Check sheet for the modelled part. Datum: model origin and axes. Units: mm. Round coordinates to 2 decimals unless told otherwise and drop trailing zeros. Loops run counter-clockwise (first coordinate to the right, second up) from the corner with the lowest first, then second, coordinate; pieces in that order, holes last. Notation, with made-up numbers: (77, -1) - (136, -1) arc R21 ccw to (136, 5) - close; hole circle Ø3 at (63, 63.25). An arc over 180 degrees is marked (long way). Put each result on its own line as item: value. Start each with the question number.
Item 1: Material ranges on line 1 along Y through (x, z) = (0, 3.75) (3 decimals); line 2 along Y through (x, z) = (7, 6); line 3 along X through (y, z) = (6.5, 0.5), recorded low to high.
Item 2: Section check D-D, the plane x = 0. Give the number of separate pieces and of enclosed holes in the cut face, and give its area (3 significant figures).
Item 3: Section check A-A, the plane z = 3.75. Record the cut outline in (x, y) (3 decimals), and give its area (3 significant figures).
Item 4: Section check C-C, the plane y = 58.72. Record the cut outline in (x, z), and give its area (3 significant figures).
Item 5: Section check B-B, the plane y = 0. Record the cut outline in (x, z) (3 decimals), and give its area (3 significant figures).
Item 6: Gauge pin test, flat end, axial feed: pin 1 Ø1.5 at (x, y) = (-7, 0) entering from +Z. Record the tip position at first contact, or that the pin passes through.
from build123d import *

# Parameters (mm, degrees)
F0_W     = 40
F0_H     = 100
F0_R     = 1.25
F0_R_2   = 1.525
F1_DEPTH = 8
F2_DEPTH = 7
F3_DEPTH = 5
F4_SIZE  = 0.99999


# Not quite as in the source:
# - a fillet or chamfer is up to 0.001 mm smaller than in the source, because OpenCascade refuses the exact size


with BuildPart() as f1:
    # F0 (on Top) → F1 (new body)
    with BuildSketch(Plane.XY):
        with Locations((0, 30)):
            Rectangle(F0_W, F0_H)
        with Locations((-7, 0)):
            Circle(F0_R, mode=Mode.SUBTRACT)
        Circle(F0_R_2, mode=Mode.SUBTRACT)
        with Locations((7, 0)):
            Circle(F0_R, mode=Mode.SUBTRACT)
        with BuildLine():
            ThreePointArc((-10.75, 30), (-10.1642135624, 31.4142135624), (-8.75, 32))
            Line((-8.75, 32), (8.75, 32))
            ThreePointArc((8.75, 32), (10.1642135624, 31.4142135624), (10.75, 30))
            Line((10.75, 30), (10.75, 11.6))
            Line((10.75, 11.6), (10.75, 5.5))
            ThreePointArc((10.75, 5.5), (8.75, 3.5), (6.75, 5.5))
            Line((6.75, 5.5), (-6.75, 5.5))
            ThreePointArc((-6.75, 5.5), (-8.75, 3.5), (-10.75, 5.5))
            Line((-10.75, 5.5), (-10.75, 11.6))
            Line((-10.75, 11.6), (-10.75, 30))
        make_face(mode=Mode.SUBTRACT)
        with BuildLine():
            Line((-1.53, 57.72), (-1.53, 59.72))
            ThreePointArc((-1.53, 59.72), (0, 61.25), (1.53, 59.72))
            Line((1.53, 59.72), (1.53, 57.72))
            ThreePointArc((1.53, 57.72), (0, 56.19), (-1.53, 57.72))
        make_face(mode=Mode.SUBTRACT)
        with Locations((7, 58.72)):
            Circle(F0_R, mode=Mode.SUBTRACT)
        with BuildLine():
            Line((8.75, 32), (-8.75, 32))
            ThreePointArc((-8.75, 32), (-10.1642135624, 31.4142135624), (-10.75, 30))
            Line((-10.75, 30), (-10.75, 11.6))
            ThreePointArc((-10.75, 11.6), (-10.1642135624, 10.1857864376), (-8.75, 9.6))
            Line((-8.75, 9.6), (8.75, 9.6))
            ThreePointArc((8.75, 9.6), (10.1642135624, 10.1857864376), (10.75, 11.6))
            Line((10.75, 11.6), (10.75, 30))
            ThreePointArc((10.75, 30), (10.1642135624, 31.4142135624), (8.75, 32))
        make_face()
        with BuildLine():
            ThreePointArc((-6, 26.3), (-5.4142135624, 27.7142135624), (-4, 28.3))
            Line((-4, 28.3), (4, 28.3))
            ThreePointArc((4, 28.3), (5.4142135624, 27.7142135624), (6, 26.3))
            Line((6, 26.3), (6, 15.3))
            ThreePointArc((6, 15.3), (5.4142135624, 13.8857864376), (4, 13.3))
            Line((4, 13.3), (-4, 13.3))
            ThreePointArc((-4, 13.3), (-5.4142135624, 13.8857864376), (-6, 15.3))
            Line((-6, 15.3), (-6, 26.3))
        make_face(mode=Mode.SUBTRACT)
        with BuildLine():
            ThreePointArc((-8.75, 9.6), (-10.1642135624, 10.1857864376), (-10.75, 11.6))
            Line((-10.75, 11.6), (-10.75, 5.5))
            ThreePointArc((-10.75, 5.5), (-8.75, 3.5), (-6.75, 5.5))
            Line((-6.75, 5.5), (6.75, 5.5))
            ThreePointArc((6.75, 5.5), (8.75, 3.5), (10.75, 5.5))
            Line((10.75, 5.5), (10.75, 11.6))
            ThreePointArc((10.75, 11.6), (10.1642135624, 10.1857864376), (8.75, 9.6))
            Line((8.75, 9.6), (-8.75, 9.6))
        make_face()
    extrude(amount=F1_DEPTH)

    # F0 (on Top) → F2 (cut)
    with BuildSketch(Plane.XY):
        with BuildLine():
            Line((8.75, 32), (-8.75, 32))
            ThreePointArc((-8.75, 32), (-10.1642135624, 31.4142135624), (-10.75, 30))
            Line((-10.75, 30), (-10.75, 11.6))
            ThreePointArc((-10.75, 11.6), (-10.1642135624, 10.1857864376), (-8.75, 9.6))
            Line((-8.75, 9.6), (8.75, 9.6))
            ThreePointArc((8.75, 9.6), (10.1642135624, 10.1857864376), (10.75, 11.6))
            Line((10.75, 11.6), (10.75, 30))
            ThreePointArc((10.75, 30), (10.1642135624, 31.4142135624), (8.75, 32))
        make_face()
        with BuildLine():
            ThreePointArc((-6, 26.3), (-5.4142135624, 27.7142135624), (-4, 28.3))
            Line((-4, 28.3), (4, 28.3))
            ThreePointArc((4, 28.3), (5.4142135624, 27.7142135624), (6, 26.3))
            Line((6, 26.3), (6, 15.3))
            ThreePointArc((6, 15.3), (5.4142135624, 13.8857864376), (4, 13.3))
            Line((4, 13.3), (-4, 13.3))
            ThreePointArc((-4, 13.3), (-5.4142135624, 13.8857864376), (-6, 15.3))
            Line((-6, 15.3), (-6, 26.3))
        make_face(mode=Mode.SUBTRACT)
    extrude(amount=F2_DEPTH, mode=Mode.SUBTRACT)

    # F0 (on Top) → F3 (cut)
    with BuildSketch(Plane.XY):
        with BuildLine():
            ThreePointArc((-8.75, 9.6), (-10.1642135624, 10.1857864376), (-10.75, 11.6))
            Line((-10.75, 11.6), (-10.75, 5.5))
            ThreePointArc((-10.75, 5.5), (-8.75, 3.5), (-6.75, 5.5))
            Line((-6.75, 5.5), (6.75, 5.5))
            ThreePointArc((6.75, 5.5), (8.75, 3.5), (10.75, 5.5))
            Line((10.75, 5.5), (10.75, 11.6))
            ThreePointArc((10.75, 11.6), (10.1642135624, 10.1857864376), (8.75, 9.6))
            Line((8.75, 9.6), (-8.75, 9.6))
        make_face()
    extrude(amount=F3_DEPTH, mode=Mode.SUBTRACT)

    # F4 (size 1 in the source; OpenCascade refuses exactly that, so slightly less here)
    f4_edges = [f1.edges().sort_by_distance(p)[0] for p in [
        (6, 20.8, 8),
        (5.414214, 13.885786, 8),
        (0, 13.3, 8),
        (-5.414214, 13.885786, 8),
        (-6, 20.8, 8),
        (-5.414214, 27.714214, 8),
        (0, 28.3, 8),
        (5.414214, 27.714214, 8),
    ]]
    chamfer(f4_edges, length=F4_SIZE)


solid = f1.part
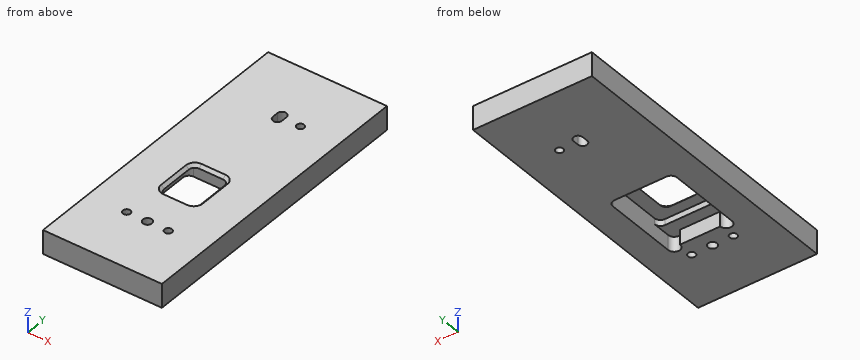
Check result:
1. line 1: -20 to -1.525, 1.525 to 5.5, 32 to 56.19, 61.25 to 80
1. line 2: -20 to -1.25, 1.25 to 9.6, 32 to 57.47, 59.97 to 80
1. line 3: -20 to -10.75, 10.75 to 20
2. separate pieces: 4
2. enclosed holes: 0
2. area: 542 mm²
3. outline: (-20, -20) - (20, -20) - (20, 80) - (-20, 80) - close; hole (-10.75, 5.5) arc R2 ccw to (-6.75, 5.5) - (6.75, 5.5) arc R2 ccw to (10.75, 5.5) - (10.75, 30) arc R2 ccw to (8.75, 32) - (-8.75, 32) arc R2 ccw to (-10.75, 30) - close; hole circle Ø2.5 at (-7, 0); hole (-1.53, 57.72) arc R1.53 ccw to (1.53, 57.72) - (1.53, 59.72) arc R1.53 ccw to (-1.53, 59.72) - close; hole circle Ø3.05 at (0, 0); hole circle Ø2.5 at (7, 0); hole circle Ø2.5 at (7, 58.72)
3. area: 3,380 mm²
4. outline: (-20, 0) - (-1.53, 0) - (-1.53, 8) - (-20, 8) - close; (1.53, 0) - (5.75, 0) - (5.75, 8) - (1.53, 8) - close; (8.25, 0) - (20, 0) - (20, 8) - (8.25, 8) - close
4. area: 276 mm²
5. outline: (-20, 0) - (-8.25, 0) - (-8.25, 8) - (-20, 8) - close; (-5.75, 0) - (-1.525, 0) - (-1.525, 8) - (-5.75, 8) - close; (1.525, 0) - (5.75, 0) - (5.75, 8) - (1.525, 8) - close; (8.25, 0) - (20, 0) - (20, 8) - (8.25, 8) - close
5. area: 256 mm²
6. pin 1: through
